Design review of the part built by this model. Coordinates are the model's own, in mm. Face numbers are marked on the shaded views. A direction names the side the tool comes from. Coordinates: 2 decimals unless noted, no trailing zeros. Loops run counter-clockwise (first coordinate to the right, second up) from the corner with the lowest first, then second, coordinate; pieces in that order, holes last. Notation, with made-up numbers: (-16.5, 60.25) - (42.5, 60.25) arc R24 ccw to (42.5, 73.25) - close; hole circle Ø5 at (-31.75, 75). An arc over 180 degrees is marked (long way). Answer in a Markdown table with one row per item. Add a question column.
(1) We need section C-C, the plane z = 3.75. Write out the cut boundary in (x, y).
(2) To check wall thickness, follow L1, parallel to Z at x = -0.3, y = 0; L2, parallel to Z at x = 0.05, y = 0; L3, parallel to X at y = -2.75, z = -3. State the ranges of each line that lie inside material, in increasing order. Write a range as [from, to].
(3) We need section B-B, the plane x = 6.5. Write out the cut boundary in (y, z), plus the area to 3 significant figures.
(4) We need section A-A, the plane x = -2. Write out the cut boundary in (y, z), plus the area to 3 significant figures.
(5) We need section D-D, the plane y = 2.75. Write out the cut boundary in (x, z).
(6) The part is to be moulded in two halves that separate along Y. For the marked faces 4, 5 and 6, say which applies: released by +Y, released by -Y, zero draft, split by the parting line, or undercut.
(7) For the marked faces 1, 2 and 3, list the 3-axis set-ups (+Z, -Z, +X, -X, +Y, -Y) from which the entire face can be reached by the end or side of a thin tool; tool diameter is ignored.
(8) Clearance check with flat-ended pins moving along their axes: pin 1 (1 mm diameter, centred on x = 5.5, z = 2.5, fed in from -Y); pin 2 (5 mm diameter, centred on y = 0.5, z = -1.5, fed in from -X); pin 3 (3 mm diameter, centred on x = 3, z = 1, fed in from +Y). State where each tip first meets the part, or that it passes through.
Autodesk Inventor part; units mm, degrees
ref_plane "Work Plane1" through (5, 0, 0) normal (0, 0.5, 0.8660254) x (1, 0, 0)
ref_plane "YZ Plane" through (0, 0, 0) normal (1, 0, 0) x (0, 1, 0)
ref_plane "XZ Plane" through (0, 0, 0) normal (0, 1, 0) x (-1, 0, 0)
sketch "草圖1" plane through (0, 0, 0) normal (0, 0, 1) x (1, 0, 0)
  line L0 (1.2217, 0) -> (10, 0)
  line L1 (10, 0) -> (10, 2.5)
  line L2 (10, 2.5) -> (0, 2.5)
  line L3 (0, 2.5) -> (0, 4.25)
  line L4 (0, 4.25) -> (-3.5, 4.25)
  line L5 (-3.5, 4.25) -> (-3.5, 2.3094)
  line L6 (-3.5, 2.3094) -> (-1.5, 2.3094)
  line L7 (-1.5, 2.3094) -> (-0.8884, 1.25)
  line L8 (-6.2, 0) -> (12.7, 0)
  line L9 (0, -0.85) -> (0, 5.1)
  line L10 (-0.8884, 1.25) -> (0.5, 1.25)
  line L11 (0.5, 1.25) -> (1.2217, 0)
  line L12 (-3.5, 2.3094) -> (-3.5, 0) construction
  dimension "d0" = 3.5
  dimension "d1" = 2
  dimension "d2" = 60
  dimension "d3" = 5
  dimension "d4" = 4.6188
  dimension "d5" = 8.5
  dimension "d15" = 4
  dimension "d16" = 2.5
  dimension "d17" = 10
revolve "本體" add sketch "草圖1" angle 360 about axis through (1.2217, 0, 0) along (1, 0, 0) contours L11 L10 L9 L2 L1 L0 | L10 L7 L6 L5 L4 L3 L9
sketch "草圖2" plane through (-3.5, 0, 0) normal (-1, 0, 0) x (0, 0, 1)
  circle A0 centre (0, 0) radius 2.3094
  line L0 (0, -5.95) -> (0, 5.95)
  line L1 (-5.95, 0) -> (5.95, 0)
  line L2 (2.3094, 0) -> (1.1547, -2)
  line L3 (1.1547, -2) -> (-1.1547, -2)
  line L4 (-1.1547, -2) -> (-2.3094, 0)
  line L5 (-2.3094, 0) -> (-1.1547, 2)
  line L6 (-1.1547, 2) -> (1.1547, 2)
  line L7 (1.1547, 2) -> (2.3094, 0)
extrude "塞槽" add sketch "草圖2" against normal up to next contours L7 A0 | A0 L2 | L6 L0 A0 | A0 L0 L3 | L0 L6 A0 | A0 L3 L0 | L4 A0 | A0 L5
thread "螺紋"
chamfer "倒角1" distance 0.4908 distance2 0.4908 1 edges at (10, -2.5, 0) measured on face at (10, -0.7741, -0.6858)
ref_plane "Work Plane1" through (5, 0, 0) normal (0, 0.5, 0.8660254) x (1, 0, 0)
equation "\"d7\" = GEL"
equation "\"d9\" = -0.5 * SPD + 0.5 * GD"
equation "\"d12\" = GUL"
equation "\"d0\" = KOH"
equation "\"d1\" = INTI"
equation "\"d3\" = GD"
equation "\"d4\" = 1.1547 * SW"
equation "\"d5\" = KOD"
equation "\"d15\" = INFT"
equation "\"d16\" = SDT"
equation "\"d17\" = NLG"
equation "\"GD\" = NND"
equation "\"NLG\" = 10"
equation "\"GEL\" = 7.4"
equation "\"KOD\" = 8.5"
equation "\"KOH\" = 3.5"
equation "\"GUL\" = 0.61345 * PTC"
equation "\"SW\" = 4"
equation "\"INTI\" = 2"
equation "\"SPD\" = NND - 1.2269 * PTC"
equation "\"SDT\" = 2.5"
equation "\"INFT\" = 4"
equation "\"TOA\" = 30deg"
equation "\"GD1\" = THREADDIA - 1.2269 * PTC"
equation "\"THREADDIA\" = 5"
equation "\"BDM\" = NND"
equation "\"RR\" = 0.5"
equation "\"PTC\" = 0.8"
equation "\"NND\" = 5"
equation "\"SLG\" = 2.6"
equation "\"GAL\" = 0.61345 * PTC"
equation "\"E0\" = 1.155 * SW"
properties part number "CNS 4557 - M5 x 10" material "鋼、軟鋼"
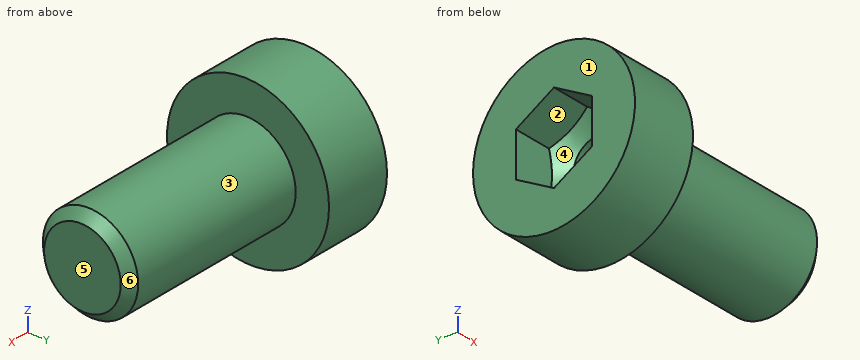
Responses:
| question | item | result |
|---|---|---|
| 1 | outline | (-3.5, -2) - (0, -2) - (0, 2) - (-3.5, 2) - close |
| 2 | L1 | z = [-4.25, -1.25], [1.25, 4.25] |
| 2 | L2 | z = [-2.5, -1.25], [1.25, 2.5] |
| 2 | L3 | x = [-3.5, 0] |
| 3 | outline | circle Ø5 at (0, 0) |
| 3 | area | 19.6 mm2 |
| 4 | outline | circle Ø8.5 at (0, 0); hole (-2, -1.15) - (0, -2.31) - (2, -1.15) - (2, 1.15) - (0, 2.31) - (-2, 1.15) - close |
| 4 | area | 42.9 mm2 |
| 5 | outline | (-3.5, -3.24) - (0, -3.24) - (0, 3.24) - (-3.5, 3.24) - close |
| 6 | face 4 | undercut |
| 6 | face 5 | zero draft |
| 6 | face 6 | split by the parting line |
| 7 | face 1 | +Z, -Z, -X, +Y, -Y |
| 7 | face 2 | -X |
| 7 | face 3 | +X |
| 8 | pin 1 | stops at y = -1.5 |
| 8 | pin 2 | stops at x = -3.5 |
| 8 | pin 3 | stops at y = 2.5 |
